```python
from build123d import *

# Parameters (mm, degrees)
F1_DEPTH = 6
F2_R     = 1.6
F3_DEPTH = 3.7
F5_SIZE2 = 2
F5_SIZE  = 2
F6_DEPTH = 2.8


with BuildPart() as f1:
    # F0 (on Front) → F1 (new body, symmetric)
    with BuildSketch(Plane.XZ):
        Polygon((-4.75, 0), (0, 0), (4.75, 0), (4.75, 3.7), (-4.75, 3.7), align=None)
    extrude(amount=F1_DEPTH, both=True)

    # F2 (on face) → F3 (cut, through all)
    with BuildSketch(Plane.XY.offset(3.7)):
        Circle(F2_R)
    extrude(amount=-F3_DEPTH, mode=Mode.SUBTRACT)

    # F5
    f5_edges = [f1.edges().sort_by_distance(p)[0] for p in [
        (-4.75, 0, 3.7),
        (4.75, 0, 3.7),
    ]]
    chamfer(f5_edges, length=F5_SIZE, length2=F5_SIZE2)

    # F4 (on face) → F6 (cut)
    with BuildSketch(Plane.XY.offset(3.7)):
        Polygon((4, -2.309401), (4, 2.309401), (0, 4.618802), (-4, 2.309401), (-4, -2.309401), (0, -4.618802), align=None)
    extrude(amount=-F6_DEPTH, mode=Mode.SUBTRACT)


solid = f1.part
```
Here's how the part is built. I have some questions about the finished solid (model axes, mm). A direction names the side the tool comes from. Coordinates: 2 decimals unless noted, no trailing zeros. Loops run counter-clockwise (first coordinate to the right, second up) from the corner with the lowest first, then second, coordinate; pieces in that order, holes last. Notation, with made-up numbers: (63, -11) - (110, -11) arc R28 ccw to (110, 24) - close; hole circle Ø4 at (-17, -7). An arc over 180 degrees is marked (long way). Return JSON: item names as keys, results as strings. Group by question number.
Item 1: Will this pin go through, and if not, where does the flat tip stop? P1, Ø3.5, axis at x = 0, y = 0, coming from the +Z side.
Item 2: On a 3-axis mill with a long thin cutter (end or side, diameter ignored), from which of +Z, -Z, +X, -X, +Y, -Y can I reach the whole of each face in a straight line? I mean faces 4 (the face through (-2.028, -3.448, 2.32)), 5 (the face through (0, -6, 2)). Say none if no direction works.
Item 3: If we section it at A-A on y = 0: Write out the boundary of the cut face in (x, z).
Item 4: I need wall thicknesses on line 1 (Y direction, x = 0, z = 0.3); line 2 (Z direction, x = 0.5, y = -2.25); line 3 (Y direction, x = -3, z = 1.4). Which ranges of each line are inside material? Lowest first, please. Write a range as from..to.
Item 5: If we section it at B-B on x = 0.5: Write out the boundary of the cut face in (y, z).
Item 6: We'd pull the mould along Y, two halves only. Please class faces 1 (the face through (-1.27, -0.97, 0.46)), 2 (the face through (4.18, 0.08, 2.27)), 3 (the face through (0, 6, 2)): +Y half, -Y half, draft (parallel to the pull), parting line (faces both ways), or undercut.
Item 7: If we section it at D-D on y = 3.25: Write out the boundary of the cut face in (x, z), and give its area (3 significant figures).
Item 8: If we section it at C-C on z = 0.3: Write out the boundary of the cut face in (x, y), and give its area (3 significant figures).
Calculated:
{
 "1": {"P1": "stops at z = 0.9"},
 "2": {"face 4": "+Z", "face 5": "+Z, -Z, +X, -X, -Y"},
 "3": {"outline": "(-4.75, 0) - (-1.6, 0) - (-1.6, 0.9) - (-4, 0.9) - (-4, 2.45) - (-4.75, 1.7) - close; (1.6, 0) - (4.75, 0) - (4.75, 1.7) - (4, 2.45) - (4, 0.9) - (1.6, 0.9) - close"},
 "4": {"line 1": "y = -6..-1.6, 1.6..6", "line 2": "z = 0..0.9", "line 3": "y = -6..-2.89, 2.89..6"},
 "5": {"outline": "(-6, 0) - (-1.52, 0) - (-1.52, 0.9) - (-4.33, 0.9) - (-4.33, 3.7) - (-6, 3.7) - close; (1.52, 0) - (6, 0) - (6, 3.7) - (4.33, 3.7) - (4.33, 0.9) - (1.52, 0.9) - close"},
 "6": {"face 1": "undercut", "face 2": "draft", "face 3": "+Y half"},
 "7": {"outline": "(-4.75, 0) - (4.75, 0) - (4.75, 1.7) - (2.75, 3.7) - (2.37, 3.7) - (2.37, 0.9) - (-2.37, 0.9) - (-2.37, 3.7) - (-2.75, 3.7) - (-4.75, 1.7) - close", "area": "17.9 mm^2"},
 "8": {"outline": "(-4.75, -6) - (4.75, -6) - (4.75, 6) - (-4.75, 6) - close; hole circle Ø3.2 at (0, 0)", "area": "106 mm^2"}
}
